Autodesk Fusion 360 part; units mm, degrees
sketch "Sketch1" plane through (0, 0, 0) normal (0, 1, 0) x (1, 0, 0)
  line L0 (0, 0) -> (101.6, 0)
  line L1 (0, 0) -> (0, -25.4)
  spline S0 degree 2 poles (0, -25.4) (61.2882, -18.6006) (101.6, 0) knots 0 0 0 10.537877 10.537877 10.537877 weights 1 2.365825 1
  spline S1 degree 2 poles (0, -20) (59.3611, -12.7) (94.0715, 0) knots 0 0 0 9.650073 9.650073 9.650073 weights 1 3 1
  dimension "d1" = 101.6
  dimension "d2" = 25.4
extrude "Extrude1" add sketch "Sketch1" along normal blind 5.08 makes body 1
extrude "Extrude2" add sketch "Sketch1" along normal blind 177.8 separate body contours L0 L1 S0 S1 makes body 2
extrude "Extrude3" add sketch "Sketch1" along normal blind 5.08 from surface at 172.72 separate body makes body 3
sketch "Sketch2" plane through (0, 0, 0) normal (0, 0, 1) x (1, 0, 0)
  line L0 (0.4808, 187.96) -> (111.76, 187.96)
  line L1 (111.76, 187.96) -> (111.76, -10.16)
  line L2 (111.76, -10.16) -> (0.4808, -10.16)
  line L3 (0.4808, -10.16) -> (0.4808, 187.96)
  line L4 (0, 0) -> (0, 177.8)
  line L5 (0, 177.8) -> (101.6, 177.8)
  line L6 (101.6, 0) -> (101.6, 177.8)
  line L7 (0, 0) -> (101.6, 0)
  circle A0 centre (97.9777, -5.1517) radius 2.4447
  line L8 (56.1204, -10.16) -> (56.1204, 187.96) construction
  line L9 (111.76, 88.9) -> (0.4808, 88.9) construction
  circle A1 centre (14.2631, -5.1517) radius 2.4447
  circle A2 centre (97.9777, 182.9517) radius 2.4447
  circle A3 centre (14.2631, 182.9517) radius 2.4447
  dimension "d13" = 10.16
  dimension "d14" = 10.16
  dimension "d15" = 10.16
  dimension "d16" = 4.8895
extrude "Extrude4" add sketch "Sketch2" along normal blind 5.08 separate body contours L0 L1 L2 L3 L5 L6 L7 makes body 4
combine "Combine1" operation add target body 3 tool bodies 4 1 2
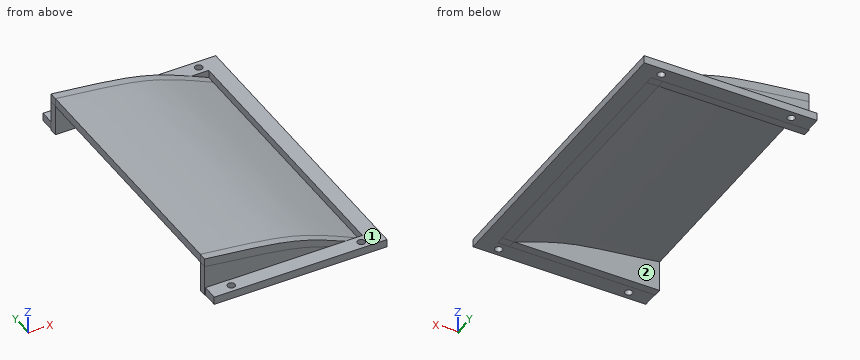
Verification items for the finished model (mm, model axes). Face numbers are marked on the shaded views. Round coordinates to 2 decimals unless told otherwise and drop trailing zeros. Write each loop counter-clockwise with the first axis right and the second up, starting at its lowest first coordinate (ties: lowest second). Pieces come first, ordered by that corner, then holes. Notation, with made-up numbers: (85.5, -17) -> (90.5, -17) arc R30 cw to (90.5, 20) -> close; hole circle Ø4 at (23.25, 88.25). An arc over 180 degrees is marked (long way). Write each question's results on one line, items separated by ' | '. Start each with the question number.
1. Depth check by flat-ended pin: P1, Ø5.5, axis at x = 97.98, y = 182.95, coming from the +Z side; P2, Ø10, axis at x = 60, z = 17, coming from the +Y side; P3, Ø2.5, axis at y = 181, z = 1.5, coming from the -X side; P4, Ø6.5, axis at x = 14.26, y = -5.15, coming from the -Z side. Enter the tip coordinate at first touch or a pass-through.
2. Material ranges on probe 1 along Y at (x, z) = (98, 4.5); probe 2 along Y at (x, z) = (77.5, 3); probe 3 along Y at (x, z) = (57, 10.25), recorded low to high. Write a range as from..to.
3. Cross-section at A-A (x = 104.5). Enter the section's corners in (y, z).
4. Draft check along Y on the marked faces 1 and 2. Enter one of: +Y half, -Y half, draft (parallel to the pull), parting line (faces both ways), or undercut.
Solutions:
1) P1: stops at z = 5.08 | P2: stops at y = 177.8 | P3: stops at x = 0.48 | P4: stops at z = 0
2) probe 1: y = -10.16..-7.6, -2.71..0, 177.8..180.51, 185.4..187.96 | probe 2: y = -10.16..5.08, 172.72..187.96 | probe 3: y = 0..5.08, 172.72..177.8
3) outline: (-10.16, 0) -> (187.96, 0) -> (187.96, 5.08) -> (-10.16, 5.08) -> close
4) face 1: draft | face 2: undercut
